Model file for the job. Use its own axes, mm. Round coordinates to 2 decimals unless told otherwise and drop trailing zeros. Write each loop counter-clockwise with the first axis right and the second up, starting at its lowest first coordinate (ties: lowest second). Pieces come first, ordered by that corner, then holes. Notation, with made-up numbers: (33, -12) - (78, -12) arc R23 ccw to (78, -3) - close; hole circle Ø9 at (-21, -6). An arc over 180 degrees is marked (long way). Answer as a JSON object with one key per item and string values. Group by question number.
from build123d import *


with BuildPart() as f1:
    # F0 (on Right) → F1 (revolve)
    with BuildSketch(Plane.YZ):
        with BuildLine():
            ThreePointArc((189.750242, 19.945681), (174.871267, 55.866706), (138.950242, 70.745681))
            Line((138.950242, 70.745681), (-140.449758, 70.745681))
            ThreePointArc((-140.449758, 70.745681), (-176.370782, 55.866706), (-191.249758, 19.945681))
            Line((-191.249758, 19.945681), (-191.249758, -30.854319))
            ThreePointArc((-191.249758, -30.854319), (-176.370782, -66.775343), (-140.449758, -81.654319))
            Line((-140.449758, -81.654319), (138.950242, -81.654319))
            ThreePointArc((138.950242, -81.654319), (174.871267, -66.775343), (189.750242, -30.854319))
            Line((189.750242, -30.854319), (189.750242, 19.945681))
        make_face()
    revolve(axis=Axis((0, -0.749758, -589.654319), (0, -1, 0)))


solid = f1.part
(1) Flat gauge pins, fed straight in: pin 1 (6 mm diameter, centred on x = -516, z = -505, fed in from -Y); pin 2 (1.5 mm diameter, centred on x = -281.5, y = -139.5, fed in from +Z); pin 3 (2 mm diameter, centred on x = 125, y = 148.5, fed in from -Z). Where does each tip first touch, or does it go through?
(2) Drill centre lines: line 1 (Z direction, x = 0, y = 36); line 2 (X direction, y = 126, z = -589); line 3 (X direction, y = 116, z = -132). Where is each one in solid material? Low to high. Write a range as from..to.
(3) Pull direction X, two halves, no side cores. Call faces 1 (the cylindrical face through (194.567, 1.206, -120.391)), 2 (the cylindrical face through (401.84, -2.71, -1113.73)), 3 (the flat face through (494, 189.75, -858)): pulls with the +X half, pulls with the -X half, needs draft (parallel to the pull), parting line crosses it, or undercut.
(4) Slice it at B-B (y = -8.5). Write the cut outline in (x, z).
(5) Slice it at A-A (x = 0). Write the cut outline in (y, z).
Answer:
{
 "1": {"pin 1": "y = -179.16", "pin 2": "z = 8.1", "pin 3": "z = -1237.46"},
 "2": {"line 1": "-1250.05..-1097.65, -81.65..70.75", "line 2": "-660.4..-508, 508..660.4", "line 3": "-476.11..-220.49, 220.49..476.11"},
 "3": {"face 1": "undercut", "face 2": "parting line crosses it", "face 3": "needs draft"},
 "4": {"outline": "circle Ø1320.8 at (0, -589.65); hole circle Ø1016 at (0, -589.65)"},
 "5": {"outline": "(-191.25, -1199.25) arc R50.8 ccw to (-140.45, -1250.05) - (138.95, -1250.05) arc R50.8 ccw to (189.75, -1199.25) - (189.75, -1148.45) arc R50.8 ccw to (138.95, -1097.65) - (-140.45, -1097.65) arc R50.8 ccw to (-191.25, -1148.45) - close; (-191.25, -30.85) arc R50.8 ccw to (-140.45, -81.65) - (138.95, -81.65) arc R50.8 ccw to (189.75, -30.85) - (189.75, 19.95) arc R50.8 ccw to (138.95, 70.75) - (-140.45, 70.75) arc R50.8 ccw to (-191.25, 19.95) - close"}
}
